CAD build for the part. Positions are in the model's coordinates, mm. A direction names the side the tool comes from. Round coordinates to 2 decimals unless told otherwise and drop trailing zeros. Write each loop counter-clockwise with the first axis right and the second up, starting at its lowest first coordinate (ties: lowest second). Pieces come first, ordered by that corner, then holes. Notation, with made-up numbers: (84, 36) - (129, 36) arc R17 ccw to (129, 48) - close; hole circle Ø5 at (-34.75, 0.5). An arc over 180 degrees is marked (long way). Put each result on its own line as item: value. Start each with the question number.
Item 1: Drill centre lines: line 1 (Y direction, x = 0, z = 152.2); line 2 (Z direction, x = -1, y = 1); line 3 (X direction, y = 1.25, z = 151.25). Where is each one in solid material? Low to high. Write a range as from..to.
Item 2: Pin check, flat tips, straight feed: pin 1 Ø2 at (y, z) = (2.5, 159) entering from -X; pin 2 Ø2 at (y, z) = (1.5, 158) entering from -X. Stop position of each tip, or through.
Item 3: Cut at A-A (y = 0). Give the cut face in (x, z).
Item 4: 3-axis set-ups, long thin cutter, end or side, ignore diameter. For faces 4 (the flat face through (0, 0, 164)), 5 (the flat face through (0, 0, 155)): which of +Z, -Z, +X, -X, +Y, -Y reach the whole face in a straight line?
Item 5: Cut at C-C (z = 153.25). Give the cut face in (x, y), and give its area (3 significant figures).
Item 6: Mould opens along X. For faces 1 (the flat face through (1.3, -1.3, 150)), 2 (the cylindrical face through (-1.5, 0.07, 152.46)), 3 (the cylindrical face through (-3, 0, 156)) say: released by +X, released by -X, zero draft, split by the parting line, or undercut.
Item 7: Cut at D-D (z = 161.5). Give the cut face in (x, y), and give its area (3 significant figures).
```python
from build123d import *

# Parameters (mm, degrees)
CYLINDER009_R     = 1.5
CYLINDER009_DEPTH = 5
CYLINDER006_R     = 3
CYLINDER006_DEPTH = 14
FILLET_R          = 1


with BuildPart() as cylinder009:
    # Cylinder009 → Cylinder009 (new body)
    with BuildSketch(Plane.XY.offset(150)):
        Circle(CYLINDER009_R)
    extrude(amount=CYLINDER009_DEPTH)


with BuildPart() as cut005:
    # Cylinder006 → Cylinder006 (new body)
    with BuildSketch(Plane.XY.offset(150)):
        Circle(CYLINDER006_R)
    extrude(amount=CYLINDER006_DEPTH)

    # Fillet
    fillet_edges = [cut005.edges().sort_by_distance(p)[0] for p in [
        (-3, 0, 164),
    ]]
    fillet(fillet_edges, radius=FILLET_R)

    # Cut005: cut Cylinder009
    add(cylinder009.part, mode=Mode.SUBTRACT)


solid = cut005.part
```
Output values:
1. line 1: -3..-1.5, 1.5..3
1. line 2: 155..164
1. line 3: -2.73..-0.83, 0.83..2.73
2. pin 1: x = -2.6
2. pin 2: x = -2.96
3. outline: (-3, 150) - (-1.5, 150) - (-1.5, 155) - (1.5, 155) - (1.5, 150) - (3, 150) - (3, 163) arc R1 ccw to (2, 164) - (-2, 164) arc R1 ccw to (-3, 163) - close
4. face 4: +Z, +X, -X, +Y, -Y
4. face 5: -Z
5. outline: circle Ø6 at (0, 0); hole circle Ø3 at (0, 0)
5. area: 21.2 mm2
6. face 1: zero draft
6. face 2: undercut
6. face 3: split by the parting line
7. outline: circle Ø6 at (0, 0)
7. area: 28.3 mm2
